```python
from build123d import *

# Parameters (mm, degrees)
ESBO_O1_W                = 589
ESBO_O1_H                = 479
RESSALTO_EXTRUS_O1_DEPTH = 296
ESBO_O2_W                = 220
ESBO_O2_H                = 180
RESSALTO_EXTRUS_O2_DEPTH = 49.2
ESBO_O3_W                = 579
ESBO_O3_H                = 469
RESSALTO_EXTRUS_O3_DEPTH = 32.8
CORTE_EXTRUS_O1_REACH    = 537.7


with BuildPart() as part:
    # Esboço1 → Ressalto-extrusão1 (new body)
    with BuildSketch(Plane(origin=(0, 0, 0), x_dir=(1, 0, 0), z_dir=(0, 1, 0))):
        Rectangle(ESBO_O1_W, ESBO_O1_H)
    extrude(amount=RESSALTO_EXTRUS_O1_DEPTH)

    # Esboço2 → Ressalto-extrusão2 (add)
    with BuildSketch(Plane(origin=(0, 296, 0), x_dir=(1, 0, 0), z_dir=(0, 1, 0))):
        Rectangle(ESBO_O2_W, ESBO_O2_H)
    extrude(amount=RESSALTO_EXTRUS_O2_DEPTH)

    # Esboço3 → Ressalto-extrusão3 (add)
    with BuildSketch(Plane(origin=(0, 345.2, 0), x_dir=(1, 0, 0), z_dir=(0, 1, 0))):
        Rectangle(ESBO_O3_W, ESBO_O3_H)
    extrude(amount=RESSALTO_EXTRUS_O3_DEPTH)

    # Corte-extrusão1: up to this face of the body (flat: up to its plane)
    corte_extrus_o1_end = Plane(part.part.faces().sort_by_distance((0, 0, 0))[0])
    # Esboço4 → Corte-extrusão1 (cut, up to the picked face)
    with BuildSketch(Plane(origin=(0, 378, 0), x_dir=(1, 0, 0), z_dir=(0, 1, 0)), mode=Mode.PRIVATE) as corte_extrus_o1_sk1:
        with BuildLine():
            ThreePointArc((-156.665637301, -234.5), (-243.283458342, -157.700862236), (-289.5, -51.565167202))
            Line((-289.5, -51.565167202), (-289.5, -234.5))
            Line((-289.5, -234.5), (-156.665637301, -234.5))
        make_face()
    corte_extrus_o1_tool1 = split(extrude(corte_extrus_o1_sk1.sketch, amount=-CORTE_EXTRUS_O1_REACH, mode=Mode.PRIVATE), bisect_by=corte_extrus_o1_end, keep=Keep.BOTH, mode=Mode.PRIVATE)
    # Esboço4 → Corte-extrusão1 (cut, up to the picked face)
    with BuildSketch(Plane(origin=(0, 378, 0), x_dir=(1, 0, 0), z_dir=(0, 1, 0)), mode=Mode.PRIVATE) as corte_extrus_o1_sk2:
        with BuildLine():
            ThreePointArc((-289.5, 51.565167202), (-243.283458342, 157.700862236), (-156.665637301, 234.5))
            Line((-156.665637301, 234.5), (-289.5, 234.5))
            Line((-289.5, 234.5), (-289.5, 51.565167202))
        make_face()
    corte_extrus_o1_tool2 = split(extrude(corte_extrus_o1_sk2.sketch, amount=-CORTE_EXTRUS_O1_REACH, mode=Mode.PRIVATE), bisect_by=corte_extrus_o1_end, keep=Keep.BOTH, mode=Mode.PRIVATE)
    # Esboço4 → Corte-extrusão1 (cut, up to the picked face)
    with BuildSketch(Plane(origin=(0, 378, 0), x_dir=(1, 0, 0), z_dir=(0, 1, 0)), mode=Mode.PRIVATE) as corte_extrus_o1_sk3:
        with BuildLine():
            Line((289.5, 234.5), (156.665637301, 234.5))
            ThreePointArc((156.665637301, 234.5), (243.283458342, 157.700862236), (289.5, 51.565167202))
            Line((289.5, 51.565167202), (289.5, 234.5))
        make_face()
    corte_extrus_o1_tool3 = split(extrude(corte_extrus_o1_sk3.sketch, amount=-CORTE_EXTRUS_O1_REACH, mode=Mode.PRIVATE), bisect_by=corte_extrus_o1_end, keep=Keep.BOTH, mode=Mode.PRIVATE)
    # Esboço4 → Corte-extrusão1 (cut, up to the picked face)
    with BuildSketch(Plane(origin=(0, 378, 0), x_dir=(1, 0, 0), z_dir=(0, 1, 0)), mode=Mode.PRIVATE) as corte_extrus_o1_sk4:
        with BuildLine():
            Line((289.5, -234.5), (289.5, -51.565167202))
            ThreePointArc((289.5, -51.565167202), (243.283458342, -157.700862236), (156.665637301, -234.5))
            Line((156.665637301, -234.5), (289.5, -234.5))
        make_face()
    corte_extrus_o1_tool4 = split(extrude(corte_extrus_o1_sk4.sketch, amount=-CORTE_EXTRUS_O1_REACH, mode=Mode.PRIVATE), bisect_by=corte_extrus_o1_end, keep=Keep.BOTH, mode=Mode.PRIVATE)
    # Esboço4 → Corte-extrusão1 (cut, up to the picked face)
    with BuildSketch(Plane(origin=(0, 378, 0), x_dir=(1, 0, 0), z_dir=(0, 1, 0)), mode=Mode.PRIVATE) as corte_extrus_o1_sk5:
        with BuildLine():
            ThreePointArc((147.25, 239.5), (151.982646469, 237.046753946), (156.665637301, 234.5))
            Line((156.665637301, 234.5), (289.5, 234.5))
            Line((289.5, 234.5), (289.5, 51.565167202))
            ThreePointArc((289.5, 51.565167202), (293.247075515, 25.903506357), (294.5, 9.48e-07))
            Line((294.5, 9.48e-07), (294.5, 239.5))
            Line((294.5, 239.5), (147.25, 239.5))
        make_face()
    corte_extrus_o1_tool5 = split(extrude(corte_extrus_o1_sk5.sketch, amount=-CORTE_EXTRUS_O1_REACH, mode=Mode.PRIVATE), bisect_by=corte_extrus_o1_end, keep=Keep.BOTH, mode=Mode.PRIVATE)
    # Esboço4 → Corte-extrusão1 (cut, up to the picked face)
    with BuildSketch(Plane(origin=(0, 378, 0), x_dir=(1, 0, 0), z_dir=(0, 1, 0)), mode=Mode.PRIVATE) as corte_extrus_o1_sk6:
        with BuildLine():
            Line((294.5, -239.5), (294.5, 9.48e-07))
            ThreePointArc((294.5, 9.48e-07), (293.247075606, -25.903505414), (289.5, -51.565167202))
            Line((289.5, -51.565167202), (289.5, -234.5))
            Line((289.5, -234.5), (156.665637301, -234.5))
            ThreePointArc((156.665637301, -234.5), (151.982646469, -237.046753946), (147.25, -239.5))
            Line((147.25, -239.5), (294.5, -239.5))
        make_face()
    corte_extrus_o1_tool6 = split(extrude(corte_extrus_o1_sk6.sketch, amount=-CORTE_EXTRUS_O1_REACH, mode=Mode.PRIVATE), bisect_by=corte_extrus_o1_end, keep=Keep.BOTH, mode=Mode.PRIVATE)
    # Esboço4 → Corte-extrusão1 (cut, up to the picked face)
    with BuildSketch(Plane(origin=(0, 378, 0), x_dir=(1, 0, 0), z_dir=(0, 1, 0)), mode=Mode.PRIVATE) as corte_extrus_o1_sk7:
        with BuildLine():
            ThreePointArc((-289.5, -51.565167202), (-293.24707556, -25.903505885), (-294.5, 0))
            Line((-294.5, 0), (-294.5, -239.5))
            Line((-294.5, -239.5), (-147.25, -239.5))
            ThreePointArc((-147.25, -239.5), (-151.982646469, -237.046753946), (-156.665637301, -234.5))
            Line((-156.665637301, -234.5), (-289.5, -234.5))
            Line((-289.5, -234.5), (-289.5, -51.565167202))
        make_face()
    corte_extrus_o1_tool7 = split(extrude(corte_extrus_o1_sk7.sketch, amount=-CORTE_EXTRUS_O1_REACH, mode=Mode.PRIVATE), bisect_by=corte_extrus_o1_end, keep=Keep.BOTH, mode=Mode.PRIVATE)
    # Esboço4 → Corte-extrusão1 (cut, up to the picked face)
    with BuildSketch(Plane(origin=(0, 378, 0), x_dir=(1, 0, 0), z_dir=(0, 1, 0)), mode=Mode.PRIVATE) as corte_extrus_o1_sk8:
        with BuildLine():
            ThreePointArc((-156.665637301, 234.5), (-151.982646469, 237.046753946), (-147.25, 239.5))
            Line((-147.25, 239.5), (-294.5, 239.5))
            Line((-294.5, 239.5), (-294.5, 0))
            ThreePointArc((-294.5, 0), (-293.24707556, 25.903505885), (-289.5, 51.565167202))
            Line((-289.5, 51.565167202), (-289.5, 234.5))
            Line((-289.5, 234.5), (-156.665637301, 234.5))
        make_face()
    corte_extrus_o1_tool8 = split(extrude(corte_extrus_o1_sk8.sketch, amount=-CORTE_EXTRUS_O1_REACH, mode=Mode.PRIVATE), bisect_by=corte_extrus_o1_end, keep=Keep.BOTH, mode=Mode.PRIVATE)
    add(corte_extrus_o1_tool1.solids().sort_by(Axis((-251.602427, 378, 184.711706), (0, -1, 0)))[0], mode=Mode.SUBTRACT)
    add(corte_extrus_o1_tool2.solids().sort_by(Axis((-251.602427, 378, -184.711706), (0, -1, 0)))[0], mode=Mode.SUBTRACT)
    add(corte_extrus_o1_tool3.solids().sort_by(Axis((251.602427, 378, -184.711706), (0, -1, 0)))[0], mode=Mode.SUBTRACT)
    add(corte_extrus_o1_tool4.solids().sort_by(Axis((251.602427, 378, 184.711706), (0, -1, 0)))[0], mode=Mode.SUBTRACT)
    add(corte_extrus_o1_tool5.solids().sort_by(Axis((152.114505, 378, -237.29506), (0, -1, 0)))[0], mode=Mode.SUBTRACT)
    add(corte_extrus_o1_tool6.solids().sort_by(Axis((220.875, 378, 236.688545), (0, -1, 0)))[0], mode=Mode.SUBTRACT)
    add(corte_extrus_o1_tool7.solids().sort_by(Axis((-293.526909, 378, 25.93064), (0, -1, 0)))[0], mode=Mode.SUBTRACT)
    add(corte_extrus_o1_tool8.solids().sort_by(Axis((-292.311455, 378, -143.032584), (0, -1, 0)))[0], mode=Mode.SUBTRACT)


solid = part.part
```
Here's how the part is built. I have some questions about the finished solid (model axes, mm). A direction names the side the tool comes from. Give positions to 0.01 mm unless a question says otherwise; leave off trailing zeros. Write each loop counter-clockwise with the first axis right and the second up, starting at its lowest first coordinate (ties: lowest second). Pieces come first, ordered by that corner, then holes. Notation, with made-up numbers: M 79,4.25 L 116,4.25 A17 cw 116,29.25 Z; hole C -29.75,23 d3. An arc over 180 degrees is marked long. Put each result on its own line as item: value. Start each with the question number.
Item 1: I need wall thicknesses on L1, parallel to Y at x = 114, z = -144.5; L2, parallel to X at y = 332.5, z = 1; L3, parallel to X at y = 203, z = -165.5. Which ranges of each line are inside material? Lowest first, please. Write a range as from..to.
Item 2: If we section it at B-B, the plane x = 225: Write out the boundary of the cut face in (y, z).
Item 3: Thinking about a two-plate mould opening in Y: for faces 4 (the flat face through (-2, 361, -234.5)), 5 (the flat face through (-2, 320, -90)), 6 (the flat face through (-4, 378, -3)), which applies, +Y half, -Y half, draft (parallel to the pull), parting line (faces both ways), or undercut?
Item 4: If we section it at D-D, the plane y = 278: Write out the boundary of the cut face in (x, z), then the cut area to 3 significant figures.
Item 5: If we section it at A-A, the plane z = 200: Write out the boundary of the cut face in (x, y), then the cut area to 3 significant figures.
Item 6: If we section it at C-C, the plane x = 2: Write out the boundary of the cut face in (y, z), then the cut area to 3 significant figures.
Item 7: Will these pins go through, and if not, where does the flat tip stop? pin 1 (6 mm diameter, centred on x = -175, y = 277, fed in from +Z); pin 2 (10 mm diameter, centred on x = 199.5, z = -22.5, fed in from -Y); pin 3 (16.5 mm diameter, centred on y = 360, z = 19, fed in from +X); pin 4 (24.5 mm diameter, centred on y = 322, z = 6, fed in from -X).
Item 8: On a 3-axis mill with a long thin cutter (end or side, diameter ignored), from which of +Z, -Z, +X, -X, +Y, -Y can I reach the whole of each face in a straight line? I mean faces 1 (the flat face through (-4, 296, 103)), 2 (the flat face through (-2, 361, 234.5)), 3 (the flat face through (-110, 320, 1)). Say none if no direction works.
Values:
1. L1: 0..296, 345.2..378
1. L2: -110..110
1. L3: -237.4..237.4
2. outline: M 0,-180.21 L 296,-180.21 L 296,180.21 L 0,180.21 Z; M 345.2,-180.21 L 378,-180.21 L 378,180.21 L 345.2,180.21 Z
3. face 4: draft
3. face 5: undercut
3. face 6: +Y half
4. outline: M -147.25,-239.5 L 147.25,-239.5 A268.4 ccw 147.25,239.5 L -147.25,239.5 A268.4 ccw Z
4. area: 242,000 mm²
5. outline: M -205.09,0 L 205.09,0 L 205.09,296 L -205.09,296 Z; M -205.09,345.2 L 205.09,345.2 L 205.09,378 L -205.09,378 Z
5. area: 135,000 mm²
6. outline: M 0,-239.5 L 296,-239.5 L 296,-90 L 345.2,-90 L 345.2,-234.5 L 378,-234.5 L 378,234.5 L 345.2,234.5 L 345.2,90 L 296,90 L 296,239.5 L 0,239.5 Z
6. area: 166,000 mm²
7. pin 1: z = 225.28
7. pin 2: y = 0
7. pin 3: x = 289.5
7. pin 4: x = -110
8. face 1: none
8. face 2: +Z, +X, -X, +Y
8. face 3: +Z, -Z, -X
